Source: three-view drawing plus pictorial views. Frame: mm from the lowest corner of the part. Coordinates: 2 decimals unless noted, no trailing zeros. Write each loop counter-clockwise with the first axis right and the second up, starting at its lowest first coordinate (ties: lowest second). Pieces come first, ordered by that corner, then holes. Notation, with made-up numbers: M 9.25,84 L 31.25,84 A14 ccw 31.25,94 Z; hole C 58,37.5 d1. An arc over 180 degrees is marked long. Use CSV: the item, a comma, the result in double quotes.
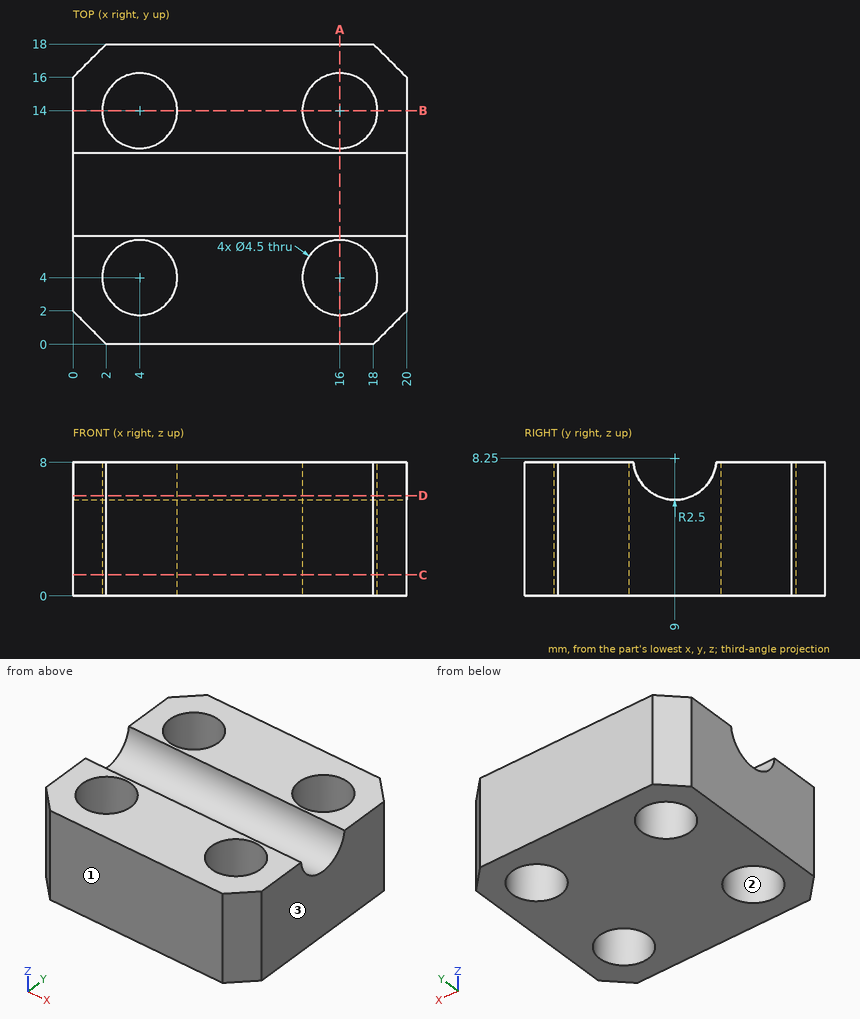
1. Section B-B (y = 14). Return loops of the section in (x, z).
Resolved:
outline,"M 0,0 L 1.75,0 L 1.75,8 L 0,8 Z; M 6.25,0 L 13.75,0 L 13.75,8 L 6.25,8 Z; M 18.25,0 L 20,0 L 20,8 L 18.25,8 Z"
2. Contact query for flat-ended pins moving along their axis: pin 1 Ø4 at (y, z) = (3, 2) entering from -X; pin 2 Ø1.5 at (x, y) = (10, 9) entering from +Z. Output: stop coordinate, or through.
Resolved:
pin 1,"stops at x = 0"
pin 2,"stops at z = 5.87"
3. Mould query, pull axis X, two halves, no side actions, for the marked faces 1, 2 and 3. Classes: pulls with the +X half, pulls with the -X half, needs draft (parallel to the pull), parting line crosses it, or undercut.
Resolved:
face 1,"needs draft"
face 2,"undercut"
face 3,"pulls with the +X half"
4. Section C-C (z = 1.25). Return loops of the section in (x, y).
Resolved:
outline,"M 0,2 L 2,0 L 18,0 L 20,2 L 20,16 L 18,18 L 2,18 L 0,16 Z; hole C 4,4 d4.5; hole C 4,14 d4.5; hole C 16,4 d4.5; hole C 16,14 d4.5"
5. Material intervals for line 1 (Y direction, x = 4, z = 4); line 2 (X direction, y = 4.5, z = 4); line 3 (Y direction, x = 4, z = 6.25), sorted ascending. Write a range as [from, to].
Resolved:
line 1,"y = [0, 1.75], [6.25, 11.75], [16.25, 18]"
line 2,"x = [0, 1.81], [6.19, 13.81], [18.19, 20]"
line 3,"y = [0, 1.75], [6.25, 7.5], [10.5, 11.75], [16.25, 18]"
6. Section A-A (x = 16). Return loops of the section in (y, z).
Resolved:
outline,"M 0,0 L 1.75,0 L 1.75,8 L 0,8 Z; M 6.25,0 L 11.75,0 L 11.75,8 L 11.49,8 A2.5 cw 6.51,8 L 6.25,8 Z; M 16.25,0 L 18,0 L 18,8 L 16.25,8 Z"
7. Section D-D (z = 6). Return loops of the section in (x, y).
Resolved:
outline,"M 0,2 L 2,0 L 18,0 L 20,2 L 20,7.91 L 0,7.91 Z; M 0,10.09 L 20,10.09 L 20,16 L 18,18 L 2,18 L 0,16 Z; hole C 4,4 d4.5; hole C 4,14 d4.5; hole C 16,4 d4.5; hole C 16,14 d4.5"
